Design review of the part shown in the three views and the two pictorial views. Dimensions are in mm from the part's minimum x, y and z. A direction names the side the tool comes from. Round coordinates to 2 decimals unless told otherwise and drop trailing zeros. Order: outer loops, then holes, each group sorted by start corner. A loop starts at its lowest first (then second) coordinate and runs counter-clockwise, first axis right, second up. Notation, with made-up numbers: (60, 74.5) - (91, 74.5) arc R30 ccw to (91, 110.5) - close; hole circle Ø4 at (75, 56.5). An arc over 180 degrees is marked (long way). One line per question, with ' | ' between items. Start each with the question number.
Item 1: Add section B-B on y = 0.85. State the section outline as (x, z) points.
Item 2: Add section A-A on z = 3.25. State the section outline as (x, y) points, and give its area (3 significant figures).
Item 3: Add section C-C on x = 10.9. State the section outline as (y, z) points.
Item 4: Tool access review of the marked faces 4, 5 and 6: name each direction out of +Z, -Z, +X, -X, +Y, -Y from which nothing blocks a thin tool from reaching the whole face with its end or side.
Item 5: For L1, parallel to X at y = 1.75, z = 3.25; L2, parallel to Z at x = 4, y = 0.55; L3, parallel to X at y = 0.2, z = 2, list the stretches that pass through material, from the lowest coordinate up. Write a range as [from, to].
Item 6: Draft analysis for pull direction X (two halves, no side actions). For the marked faces 1, 2 and 3, state which applies: +X half, -X half, draft (parallel to the pull), parting line (faces both ways), or undercut.
Item 7: Add section D-D on z = 4.5. State the section outline as (x, y) points, and give its area (3 significant figures).
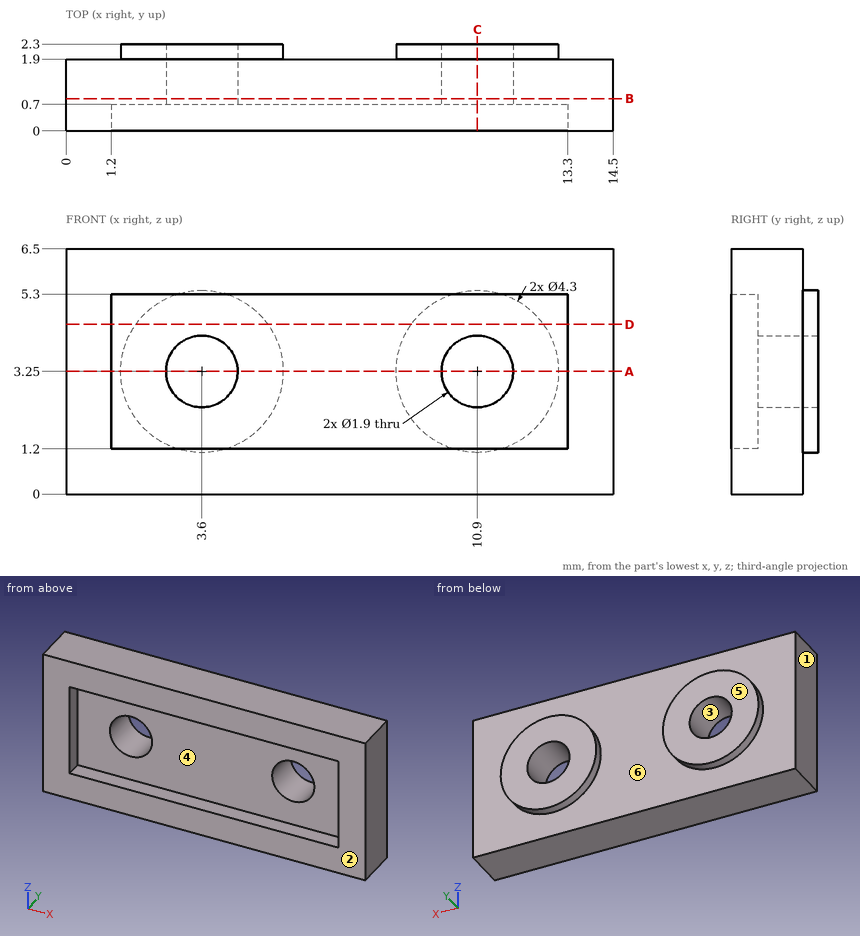
Determined:
1) outline: (0, 0) - (14.5, 0) - (14.5, 6.5) - (0, 6.5) - close; hole circle Ø1.9 at (3.6, 3.25); hole circle Ø1.9 at (10.9, 3.25)
2) outline: (0, 0) - (1.2, 0) - (1.2, 0.7) - (2.65, 0.7) - (2.65, 2.3) - (1.45, 2.3) - (1.45, 1.9) - (0, 1.9) - close; (4.55, 0.7) - (9.95, 0.7) - (9.95, 2.3) - (8.75, 2.3) - (8.75, 1.9) - (5.75, 1.9) - (5.75, 2.3) - (4.55, 2.3) - close; (11.85, 0.7) - (13.3, 0.7) - (13.3, 0) - (14.5, 0) - (14.5, 1.9) - (13.05, 1.9) - (13.05, 2.3) - (11.85, 2.3) - close | area: 16.4 mm2
3) outline: (0, 0) - (1.9, 0) - (1.9, 1.1) - (2.3, 1.1) - (2.3, 2.3) - (0.7, 2.3) - (0.7, 1.2) - (0, 1.2) - close; (0, 5.3) - (0.7, 5.3) - (0.7, 4.2) - (2.3, 4.2) - (2.3, 5.4) - (1.9, 5.4) - (1.9, 6.5) - (0, 6.5) - close
4) face 4: -Y | face 5: +Z, -Z, +X, -X, +Y | face 6: +Y
5) L1: [0, 2.65], [4.55, 9.95], [11.85, 14.5] | L2: [0, 1.2], [5.3, 6.5] | L3: [0, 1.2], [13.3, 14.5]
6) face 1: -X half | face 2: draft | face 3: undercut
7) outline: (0, 0) - (1.2, 0) - (1.2, 0.7) - (13.3, 0.7) - (13.3, 0) - (14.5, 0) - (14.5, 1.9) - (12.65, 1.9) - (12.65, 2.3) - (9.15, 2.3) - (9.15, 1.9) - (5.35, 1.9) - (5.35, 2.3) - (1.85, 2.3) - (1.85, 1.9) - (0, 1.9) - close | area: 21.9 mm2
